```python
from build123d import *

# Parameters (mm, degrees)
F0_W     = 100
F0_H     = 100
F1_DEPTH = 50
F2_R     = 93.876824
F3_DEPTH = 75


with BuildPart() as f1:
    # F0 (on Right) → F1 (new body)
    with BuildSketch(Plane.YZ):
        with Locations((27.192001, 6.234261)):
            Rectangle(F0_W, F0_H)
    extrude(amount=F1_DEPTH)


with BuildPart() as f3:
    # F2 (on Right) → F3 (new body)
    with BuildSketch(Plane.YZ):
        with Locations((-22.840602, 56.513045)):
            Circle(F2_R)
    extrude(amount=F3_DEPTH)


with BuildPart() as f1_1:
    add(f1.part)

    # F4: cut F3
    add(f3.part, mode=Mode.SUBTRACT)


solid = f1_1.part
```
CAD build for the part. Positions are in the model's coordinates, mm. Round coordinates to 2 decimals unless told otherwise and drop trailing zeros. Order: outer loops, then holes, each group sorted by start corner. A loop starts at its lowest first (then second) coordinate and runs counter-clockwise, first axis right, second up.
Item 1: Saw through at A-A on x = 43. Write the cut outline in (y, z).
Item 2: Pin check, flat tip, straight feed: pin 1 (6 mm diameter, centred on x = 37, z = -24, fed in from -Y). Stop position of the tip, or through.
Item 3: Saw through at C-C on z = 21. Write the cut outline in (x, y), then the cut area to 3 significant figures.
Item 4: Saw through at B-B on y = 5.5. Write the cut outline in (x, z), then the cut area to 3 significant figures.
Item 5: Probe line 1 along Z through (x, y) = (7.5, 55.5); line 2 along Y through (x, z) = (39, 28); line 3 along Z through (x, y) = (27.5, -2.5). List the from-to ranges inside material, lowest first.
Reported:
1. outline: (-22.81, -43.77) - (77.19, -43.77) - (77.19, 56.23) - (71.04, 56.23) arc R93.88 cw to (-22.81, -37.36) - close
2. pin 1: stops at y = 20.04
3. outline: (0, 64.06) - (50, 64.06) - (50, 77.19) - (0, 77.19) - close
3. area: 657 mm2
4. outline: (0, -43.77) - (50, -43.77) - (50, -32.98) - (0, -32.98) - close
4. area: 539 mm2
5. line 1: z = -43.77 to 4.79
5. line 2: y = 66.6 to 77.19
5. line 3: z = -43.77 to -35.13
